from build123d import *

# Parameters (mm, degrees)
F1_DEPTH = 10
F3_D     = 3.5
F3_DEPTH = 20
F3_TIP   = 1.0515060833


with BuildPart() as f1:
    # F0 (on Top) → F1 (new body)
    with BuildSketch(Plane.XY):
        Polygon((0, 0), (14, 0), (14, 5), (13, 5), (10, 5), (-10, 5), (-13, 5), (-14, 5), (-14, 0), align=None)
        with BuildLine():
            Line((10, 5), (13, 5))
            Line((13, 5), (13, 13))
            add(Edge.make_bspline(
                [(10, 13), (10.0875152242, 17.3310754155), (3.1900581528, 18.3531665627), (12.4792576098, 18.1416594137), (12.7652252364, 14.7197898641), (13, 13)],
                knots=[0, 0, 0, 0, 0.3647942323, 0.6803735299, 1, 1, 1, 1], degree=3))
            Line((10, 13), (10, 5))
        make_face()
        with BuildLine():
            Line((-13, 5), (-10, 5))
            Line((-10, 5), (-10, 13))
            add(Edge.make_bspline(
                [(-10, 13), (-10.0875152242, 17.3310754155), (-3.1900581528, 18.3531665627), (-12.4792576098, 18.1416594137), (-12.7652252364, 14.7197898641), (-13, 13)],
                knots=[0, 0, 0, 0, 0.3647942323, 0.6803735299, 1, 1, 1, 1], degree=3))
            Line((-13, 13), (-13, 5))
        make_face()
    extrude(amount=F1_DEPTH)

    # F3
    with Locations(Plane.XZ):
        with Locations((0, 4.9098548479)):
            Hole(F3_D / 2, depth=F3_DEPTH)
            with Locations((0, 0, -(F3_DEPTH + F3_TIP / 2))):  # 118° drill point
                Cone(0, F3_D / 2, F3_TIP, mode=Mode.SUBTRACT)


solid = f1.part
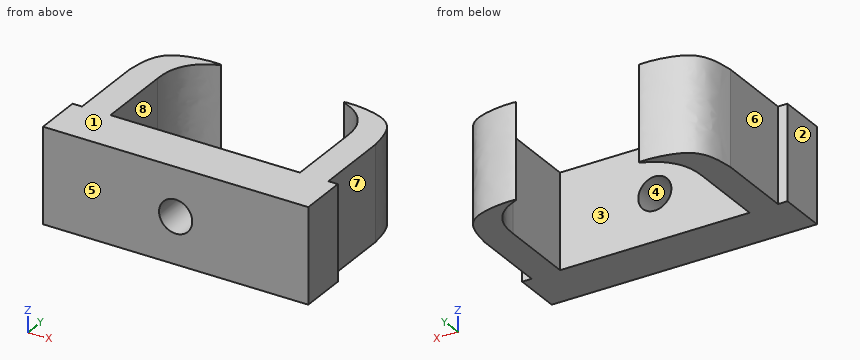
Geometry check sheet. Reference: the model listing, model coordinates, mm. Face numbers are marked on the shaded views. A direction names the side the tool comes from. Give positions to 0.01 mm unless a question says otherwise; leave off trailing zeros. Loops run counter-clockwise (first coordinate to the right, second up) from the corner with the lowest first, then second, coordinate; pieces in that order, holes last. Notation, with made-up numbers: M 44.5,74 L 95.5,74 A31 cw 95.5,113 Z; hole C 84.25,-26.75 d10. An arc over 180 degrees is marked long. Answer as a JSON object with one key per item and string values. Group by question number.
Item 1: Sectioned sample at C-C on x = -3. Record the boundary of the cut face in (y, z).
Item 2: Sectioned sample at B-B on y = 12. Record the boundary of the cut face in (x, z), plus the area to 3 significant figures.
Item 3: Sectioned sample at A-A on x = 0. Record the boundary of the cut face in (y, z), plus the area to 3 significant figures.
Item 4: Mould release check, pull along X, two halves, no side actions. Record for the marked faces 1, 2, 3 and 4: pulls with the +X half, pulls with the -X half, needs draft (parallel to the pull), parting line crosses it, or undercut.
Item 5: Gauge pin test, flat ends, axial feed: pin 1 (3 mm diameter, centred on y = 9, z = 4, fed in from -X); pin 2 (3 mm diameter, centred on x = 1.5, z = 5, fed in from +Y). Record the tip position at first contact, or that the pin passes through.
Item 6: Material ranges on L1, parallel to Z at x = 0, y = 3.4; L2, parallel to X at y = 9, z = 4.5; L3, parallel to Y at x = -5.25, z = 9.75, recorded low to high.
Item 7: Access from +Z, -Z, +X, -X, +Y, -Y to the whole of each face (thin tool, end or side, straight path). Record for the marked faces 5, 6, 7 and 8.
Findings below:
{
 "1": {"outline": "M 0,0 L 5,0 L 5,10 L 0,10 Z"},
 "2": {"outline": "M -13,0 L -10,0 L -10,10 L -13,10 Z; M 10,0 L 13,0 L 13,10 L 10,10 Z", "area": "60.0 mm2"},
 "3": {"outline": "M 0,0 L 5,0 L 5,3.16 L 0,3.16 Z; M 0,6.66 L 5,6.66 L 5,10 L 0,10 Z", "area": "32.5 mm2"},
 "4": {"face 1": "needs draft", "face 2": "pulls with the -X half", "face 3": "undercut", "face 4": "undercut"},
 "5": {"pin 1": "x = -13", "pin 2": "y = 5"},
 "6": {"L1": "0 to 3.16, 6.66 to 10", "L2": "-13 to -10, 10 to 13", "L3": "0 to 5"},
 "7": {"face 5": "+Z, -Z, +X, -X, -Y", "face 6": "+Z, -Z, -X, +Y", "face 7": "+Z, -Z, +X, +Y", "face 8": "+Z, -Z"}
}
